Print and shaded views of the part. All mm, measured from the part's lowest x, y and z. A direction names the side the tool comes from. Round coordinates to 2 decimals unless told otherwise and drop trailing zeros. Write each loop counter-clockwise with the first axis right and the second up, starting at its lowest first coordinate (ties: lowest second). Pieces come first, ordered by that corner, then holes. Notation, with made-up numbers: M 56,22 L 98,22 A12 cw 98,37 Z; hole C -14.5,50.5 d11. An arc over 180 degrees is marked long. Write item = value, one per line.
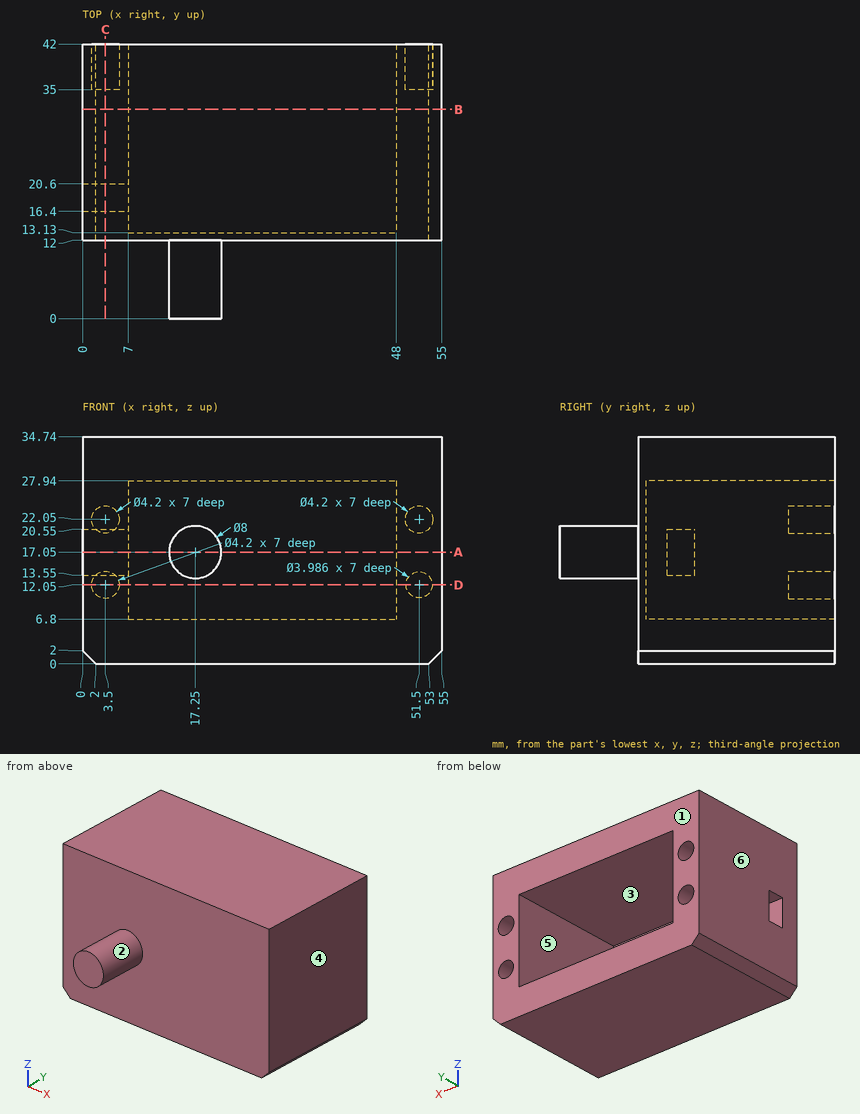
1. Band-saw the part on A-A (z = 17.05). List the corners of the cut face in (x, y).
Responses:
outline = M 0,12 L 13.25,12 L 13.25,0 L 21.25,0 L 21.25,12 L 55,12 L 55,42 L 48,42 L 48,13.13 L 7,13.13 L 7,16.4 L 0,16.4 Z; M 0,20.6 L 7,20.6 L 7,42 L 0,42 Z
2. Band-saw the part on D-D (z = 12.05). List the corners of the cut face in (x, y), plus the area to 3 significant figures.
Responses:
outline = M 0,12 L 55,12 L 55,42 L 53.49,42 L 53.49,35 L 49.51,35 L 49.51,42 L 48,42 L 48,13.13 L 7,13.13 L 7,42 L 5.6,42 L 5.6,35 L 1.4,35 L 1.4,42 L 0,42 Z
area = 409 mm²
3. Band-saw the part on B-B (y = 32). List the corners of the cut face in (x, z), plus the area to 3 significant figures.
Responses:
outline = M 0,2 L 2,0 L 53,0 L 55,2 L 55,34.74 L 0,34.74 Z; hole M 7,6.8 L 48,6.8 L 48,27.94 L 7,27.94 Z
area = 1,040 mm²
4. Tool access for the marked faces 1, 2 and 3: list every direction of +Z, -Z, +X, -X, +Y, -Y with a clear straight run to the whole face (end or side of a thin tool).
Responses:
face_1 = +Z, -Z, +X, -X, +Y
face_2 = -Y
face_3 = +Y
5. Band-saw the part on C-C (x = 3.5). List the corners of the cut face in (y, z), plus the area to 3 significant figures.
Responses:
outline = M 12,0 L 42,0 L 42,9.95 L 35,9.95 L 35,14.15 L 42,14.15 L 42,19.95 L 35,19.95 L 35,24.15 L 42,24.15 L 42,34.74 L 12,34.74 Z; hole M 16.4,13.55 L 20.6,13.55 L 20.6,20.55 L 16.4,20.55 Z
area = 954 mm²
6. Mould opens along X. For the marked faces 4, 5 and 6 say: pulls with the +X half, pulls with the -X half, needs draft (parallel to the pull), parting line crosses it, or undercut.
Responses:
face_4 = pulls with the +X half
face_5 = undercut
face_6 = pulls with the -X half
7. Flat gauge pins, fed straight in: pin 1 (7.5 mm diameter, centred on x = 2, z = 16, fed in from -Y); pin 2 (2 mm diameter, centred on x = 51, z = 22.5, fed in from +Y). Where does each tip first touch, or does it go through?
Responses:
pin_1 = 12
pin_2 = 35
8. Probe probe 1 along Z at (x, y) = (3.5, 40); probe 2 along X at (y, z) = (39, 22); probe 3 along Z at (x, y) = (51.5, 40.25). List the from-to ranges inside material, lowest first.
Responses:
probe_1 = 0 to 9.95, 14.15 to 19.95, 24.15 to 34.74
probe_2 = 0 to 1.4, 5.6 to 7, 48 to 49.4, 53.6 to 55
probe_3 = 0 to 10.06, 14.04 to 19.95, 24.15 to 34.74
